Check sheet for the modelled part. Datum: model origin and axes. Units: mm. A direction names the side the tool comes from. Give positions to 0.01 mm unless a question says otherwise; leave off trailing zeros.
```python
from build123d import *

# Parameters (mm, degrees)
F2_R     = 2.1
F3_DEPTH = 13.001
F2_R_2   = 3.75
F4_DEPTH = 3


with BuildPart() as f1:
    # F0 (on Front) → F1 (revolve)
    with BuildSketch(Plane.XZ):
        with BuildLine():
            Line((0, -6.5), (0, 6.5))
            Line((0, 6.5), (-4.5, 6.5))
            ThreePointArc((-4.5, 6.5), (-7.905694, 0), (-4.5, -6.5))
            Line((-4.5, -6.5), (0, -6.5))
        make_face()
    revolve(axis=Axis((0, 0, 0), (0, 0, 1)))

    # F2 (on face) → F3 (cut, through all)
    with BuildSketch(Plane.XY.offset(6.5)):
        Circle(F2_R)
    extrude(amount=-F3_DEPTH, mode=Mode.SUBTRACT)

    # F2 (on face) → F4 (cut)
    with BuildSketch(Plane.XY.offset(6.5)):
        Circle(F2_R_2)
        Circle(F2_R, mode=Mode.SUBTRACT)
    extrude(amount=-F4_DEPTH, mode=Mode.SUBTRACT)


solid = f1.part
```
Q1. Material ranges on line 1 (Z direction, x = -2.5, y = 1); line 2 (Y direction, x = 0, z = -4.5); line 3 (Y direction, x = -2, z = 5.5), recorded low to high.
Q2. Draft check along X on faces 1 (the flat face through (-1, -4, 6.5)), 2 (the cylindrical face through (-3.746, 0.165, 5.021)). Enter one of: pulls with the +X half, pulls with the -X half, needs draft (parallel to the pull), parting line crosses it, or undercut.
Q3. Tool access check on faces 3 (the flat face through (2.1, 0.9, -6.5)), 4 (the flat face through (2, -2, 3.5)). Record the directions out of +Z, -Z, +X, -X, +Y, -Y that give a thin tool (end or side, any length) a straight path to the whole face; none if there is none.
Q4. Go/stop test with flat-tipped pins: P1, Ø6, axis at y = 0.5, z = -3.5, coming from the -X side; P2, Ø3, axis at y = 5, z = 2.5, coming from the +X side; P3, Ø2, axis at x = -0.5, y = -5.5, coming from the +Z side. Record where each tip stops, or that it passes through.
Filled in:
1. line 1: z = -6.5 to 3.5
1. line 2: y = -6.5 to -2.1, 2.1 to 6.5
1. line 3: y = -5.32 to -3.17, 3.17 to 5.32
2. face 1: needs draft
2. face 2: undercut
3. face 3: -Z, +X, -X, +Y, -Y
3. face 4: +Z
4. P1: stops at x = -7.89
4. P2: stops at x = 6.77
4. P3: stops at z = 6.48
